Here's how the part is built. I have some questions about the finished solid (model axes, mm). A direction names the side the tool comes from. Round coordinates to 2 decimals unless told otherwise and drop trailing zeros. Write each loop counter-clockwise with the first axis right and the second up, starting at its lowest first coordinate (ties: lowest second). Pieces come first, ordered by that corner, then holes. Notation, with made-up numbers: (62.5, -35) - (90.5, -35) arc R15 ccw to (90.5, -23) - close; hole circle Ø4 at (34.25, 72.25). An arc over 180 degrees is marked (long way). Write item = value, one per line. Start each with the question number.
Item 1: If we section it at C-C (x = -22): Please give me the cut outline in (y, z), and give its area (3 significant figures).
Item 2: If we section it at B-B (y = -8.75): Please give me the cut outline in (x, z) (3 decimals), and give its area (3 significant figures).
Item 3: For P1, Ø6, axis at x = 30.5, z = 6, coming from the -Y side; P2, Ø1.1, axis at x = 26, y = -13.5, coming from the -Z side; P3, Ø6, axis at x = -29, z = 8, coming from the -Y side; P4, Ø1.5, axis at x = -23, z = 3, coming from the -Y side, each with a flat end and sliding along its axis, tell me the tip position at first contact or that it passes through.
Item 4: If we section it at A-A (z = 6.35): Please give me the cut outline in (x, y) (3 decimals).
Item 5: Which directions (+Z, -Z, +X, -X, +Y, -Y) give clear straight access to the entire face, cutting with the end or side of a thin tool? Please do faces 1 (the face through (-38, -13, 10.16)), 2 (the face through (1, -6, 12.7)).
Item 6: If we section it at D-D (z = 1.5): Please give me the cut outline in (x, y) (3 decimals).
Item 7: If I drill on line 1 along X through (y, z) = (-5, 6.35) (3 decimals); line 2 along X through (y, z) = (-7.5, 7.75) (3 decimals); line 3 along Y through (x, z) = (-1.5, 9.5), over which ranges is the centre line in solid material (lowest first)? Write a range as [from, to].
```python
from build123d import *

# Parameters (mm, degrees)
BOSS_EXTRUDE1_DEPTH = 12.7
SKETCH2_R           = 2.5
CUT_EXTRUDE1_DEPTH  = 16.24
SKETCH3_W           = 7.62
SKETCH3_H           = 3.81
CUT_EXTRUDE2_DEPTH  = 93.1900001


with BuildPart() as part:
    # Sketch1 → Boss-Extrude1 (new body)
    with BuildSketch(Plane.XY):
        with BuildLine():
            Line((-46.095, 0), (46.095, 0))
            Line((46.095, 0), (46.095, -15.24))
            ThreePointArc((46.095, -15.24), (0, -10.796372038), (-46.095, -15.24))
            Line((-46.095, -15.24), (-46.095, 0))
        make_face()
    extrude(amount=BOSS_EXTRUDE1_DEPTH)

    # Sketch2 → Cut-Extrude1 (cut, through all)
    with BuildSketch(Plane(origin=(0, 0, 0), x_dir=(1, 0, 0), z_dir=(0, 1, 0))):
        with Locations((-39.095, -6.35)):
            Circle(SKETCH2_R)
        with Locations((39.095, -6.35)):
            Circle(SKETCH2_R)
    extrude(amount=-CUT_EXTRUDE1_DEPTH, mode=Mode.SUBTRACT)

    # Sketch3 → Cut-Extrude2 (cut, through all)
    with BuildSketch(Plane(origin=(46.095, 0, 0), x_dir=(0, 0, -1), z_dir=(1, 0, 0))):
        with Locations((-6.35, -13.335)):
            Rectangle(SKETCH3_W, SKETCH3_H)
    extrude(amount=-CUT_EXTRUDE2_DEPTH, mode=Mode.SUBTRACT)


solid = part.part
```
Reply:
q1.outline = (-11.8, 0) - (0, 0) - (0, 12.7) - (-11.8, 12.7) - (-11.8, 10.16) - (-11.43, 10.16) - (-11.43, 2.54) - (-11.8, 2.54) - close
q1.area = 147 mm2
q2.outline = (-46.095, 0) - (46.095, 0) - (46.095, 12.7) - (-46.095, 12.7) - close; hole circle Ø5 at (-39.095, 6.35); hole circle Ø5 at (39.095, 6.35)
q2.area = 1,130 mm2
q3.P1 = -11.43
q3.P2 = through
q3.P3 = -12.81
q3.P4 = -11.95
q4.outline = (-46.095, -11.43) - (-41.595, -11.43) - (-41.595, 0) - (-46.095, 0) - close; (-36.595, -11.43) - (-17.475, -11.43) arc R241.3 cw to (17.475, -11.43) - (36.595, -11.43) - (36.595, 0) - (-36.595, 0) - close; (41.595, -11.43) - (46.095, -11.43) - (46.095, 0) - (41.595, 0) - close
q5.face_1 = +X, -X, -Y
q5.face_2 = +Z, +X, -X, +Y, -Y
q6.outline = (-46.095, -15.24) arc R241.3 cw to (46.095, -15.24) - (46.095, 0) - (-46.095, 0) - close
q7.line_1 = [-46.095, -41.595], [-36.595, 36.595], [41.595, 46.095]
q7.line_2 = [-46.095, -41.166], [-37.024, 37.024], [41.166, 46.095]
q7.line_3 = [-10.8, 0]
